Geometry: final body of the model. Coordinates: model frame, mm. A direction names the side the tool comes from. Give positions to 0.01 mm unless a question says otherwise; leave off trailing zeros. Write each loop counter-clockwise with the first axis right and the second up, starting at its lowest first coordinate (ties: lowest second). Pieces come first, ordered by that corner, then holes. Notation, with made-up numbers: (-11, 1) - (25, 1) arc R12 ccw to (25, 22) - close; hole circle Ø9 at (-9, -0.75). An arc over 180 degrees is marked (long way). Return JSON: item names as keys, results as strings.
from build123d import *

# Parameters (mm, degrees)
LID_PLATE_DEPTH        = 2.4
DRIP_SKIRT_DEPTH       = 3.01
SKETCH3_W              = 25.3
SKETCH3_H              = 1.9
FRONT_SKIRT_L_DEPTH    = 5.4
SKETCH4_W              = 25.3
SKETCH4_H              = 1.9
FRONT_SKIRT_R_DEPTH    = 5.4
SKETCH5_W              = 63
SKETCH5_H              = 34
GNSS_THIN_WINDOW_DEPTH = 1.7
SKETCH6_R              = 1.7
SCREW_HOLES_DEPTH      = 4.4


with BuildPart() as part:
    # Sketch1 → Lid Plate (new body)
    with BuildSketch(Plane(origin=(0, 10, 0), x_dir=(1, 0, 0), z_dir=(0, 1, 0))):
        Polygon((-65.187005769, -156.3), (65.187005769, -156.3), (74.3, -147.187005769), (74.3, -11.9), (-74.3, -11.9), (-74.3, -147.187005769), align=None)
    extrude(amount=LID_PLATE_DEPTH)

    # Sketch2 → Drip Skirt (add)
    with BuildSketch(Plane(origin=(0, 7, 0), x_dir=(1, 0, 0), z_dir=(0, 1, 0))):
        Polygon((74.3, -11.9), (74.3, -147.187005769), (65.187005769, -156.3), (-65.187005769, -156.3), (-74.3, -147.187005769), (-74.3, -11.9), (-72.7, -11.9), (-72.7, -146.524264069), (-64.524264069, -154.7), (64.524264069, -154.7), (72.7, -146.524264069), (72.7, -11.9), align=None)
    extrude(amount=DRIP_SKIRT_DEPTH)

    # Sketch3 → Front Skirt L (add)
    with BuildSketch(Plane(origin=(0, 7, 0), x_dir=(1, 0, 0), z_dir=(0, 1, 0))):
        with Locations((-61.65, -10.95)):
            Rectangle(SKETCH3_W, SKETCH3_H)
    extrude(amount=FRONT_SKIRT_L_DEPTH)

    # Sketch4 → Front Skirt R (add)
    with BuildSketch(Plane(origin=(0, 7, 0), x_dir=(1, 0, 0), z_dir=(0, 1, 0))):
        with Locations((61.65, -10.95)):
            Rectangle(SKETCH4_W, SKETCH4_H)
    extrude(amount=FRONT_SKIRT_R_DEPTH)

    # Sketch5 → GNSS Thin Window (cut)
    with BuildSketch(Plane(origin=(0, 9.5, 0), x_dir=(1, 0, 0), z_dir=(0, 1, 0))):
        with Locations((-8.5, -123)):
            Rectangle(SKETCH5_W, SKETCH5_H)
    extrude(amount=GNSS_THIN_WINDOW_DEPTH, mode=Mode.SUBTRACT)

    # Sketch6 → Screw Holes (cut)
    with BuildSketch(Plane(origin=(0, 9, 0), x_dir=(1, 0, 0), z_dir=(0, 1, 0))):
        with Locations(Location((-66.5, -18.5, 0), (0, 0, 270))):
            Circle(SKETCH6_R)
        with Locations(Location((66.5, -18.5, 0), (0, 0, 270))):
            Circle(SKETCH6_R)
        with Locations(Location((-66.5, -91, 0), (0, 0, 270))):
            Circle(SKETCH6_R)
        with Locations(Location((66.5, -91, 0), (0, 0, 270))):
            Circle(SKETCH6_R)
        with Locations(Location((-64, -146, 0), (0, 0, 270))):
            Circle(SKETCH6_R)
        with Locations(Location((64, -146, 0), (0, 0, 270))):
            Circle(SKETCH6_R)
        with Locations(Location((-44, -24, 0), (0, 0, 270))):
            Circle(SKETCH6_R)
        with Locations(Location((-44, -80, 0), (0, 0, 270))):
            Circle(SKETCH6_R)
        with Locations(Location((44, -24, 0), (0, 0, 270))):
            Circle(SKETCH6_R)
        with Locations(Location((44, -80, 0), (0, 0, 270))):
            Circle(SKETCH6_R)
    extrude(amount=SCREW_HOLES_DEPTH, mode=Mode.SUBTRACT)


solid = part.part
Q1. Section query D-D, the plane x = -29. Return the cut outline in (y, z), plus the area to 3 significant figures.
Answer key:
{"outline": "(7, 154.7) - (10, 154.7) - (10, 140) - (11.2, 140) - (11.2, 106) - (10, 106) - (10, 11.9) - (12.4, 11.9) - (12.4, 156.3) - (7, 156.3) - close", "area": "311 mm^2"}
Q2. Set-up query: faces 1 (the flat face through (68.555, 8.479, 150.669)), 2 (the cylindrical face through (65, 11.2, 19.3)). Return all of +Z, -Z, +X, -X, +Y, -Y with unobstructed straight access to the full face (end or side cutting, diameter ignored); none if empty.
Answer key:
{"face 1": "-Y", "face 2": "+Y, -Y"}
Q3. Section query C-C, the plane y = 8.1. Return the cut outline in (x, z), plus the area to 3 significant figures.
Answer key:
{"outline": "(-74.3, 10) - (-49, 10) - (-49, 11.9) - (-72.7, 11.9) - (-72.7, 146.52) - (-64.52, 154.7) - (64.52, 154.7) - (72.7, 146.52) - (72.7, 11.9) - (49, 11.9) - (49, 10) - (74.3, 10) - (74.3, 147.19) - (65.19, 156.3) - (-65.19, 156.3) - (-74.3, 147.19) - close", "area": "775 mm^2"}
Q4. Material intervals for probe 1 along X at (y, z) = (10.95, 146); probe 2 along X at (y, z) = (10.65, 91); probe 3 along Z at (x, y) = (44, 10.75), sorted ascending. Write a range as [from, to].
Answer key:
{"probe 1": "x = [-74.3, -65.7], [-62.3, 62.3], [65.7, 74.3]", "probe 2": "x = [-74.3, -68.2], [-64.8, 64.8], [68.2, 74.3]", "probe 3": "z = [11.9, 22.3], [25.7, 78.3], [81.7, 156.3]"}
Q5. Section query B-B, the plane z = 24. Return the cut outline in (x, y).
Answer key:
{"outline": "(-74.3, 7) - (-72.7, 7) - (-72.7, 10) - (-45.7, 10) - (-45.7, 12.4) - (-74.3, 12.4) - close; (-42.3, 10) - (42.3, 10) - (42.3, 12.4) - (-42.3, 12.4) - close; (45.7, 10) - (72.7, 10) - (72.7, 7) - (74.3, 7) - (74.3, 12.4) - (45.7, 12.4) - close"}
Q6. Section query A-A, the plane x = -44. Return the cut outline in (y, z).
Answer key:
{"outline": "(7, 154.7) - (10, 154.7) - (10, 81.7) - (12.4, 81.7) - (12.4, 156.3) - (7, 156.3) - close; (10, 11.9) - (12.4, 11.9) - (12.4, 22.3) - (10, 22.3) - close; (10, 25.7) - (12.4, 25.7) - (12.4, 78.3) - (10, 78.3) - close"}
Q7. Mould query, pull axis Z, two halves, no side actions, for faces 3 (the flat face through (-68.669, 8.479, 150.555)), 4 (the cylindrical face through (-66.43, 11.18, 89.3)), 5 (the flat face through (61, 10, 10)), 6 (the flat face through (-69.68, 9.662, 151.807)). Classes: pulls with the +Z half, pulls with the -Z half, needs draft (parallel to the pull), parting line crosses it, or undercut.
Answer key:
{"face 3": "undercut", "face 4": "undercut", "face 5": "pulls with the -Z half", "face 6": "pulls with the +Z half"}
Q8. Pin query (flat end, axial travel): P1, Ø4.5, axis at x = 44, z = 24, coming from the -Y side; P2, Ø2, axis at x = 66.5, z = 91, coming from the -Y side; P3, Ø1, axis at x = -6.5, y = 11, coming from the -Z side; P4, Ø1.5, axis at x = -6.5, y = 9, coming from the -Z side. Return the tip coordinate at first contact, or that it passes through.
Answer key:
{"P1": "stops at y = 10", "P2": "passes through", "P3": "stops at z = 11.9", "P4": "stops at z = 154.7"}
